The model under review builds one solid part; all positions refer to its coordinate system, in mm. Face numbers are marked on the shaded views. A direction names the side the tool comes from. Round coordinates to 2 decimals unless told otherwise and drop trailing zeros. Loops run counter-clockwise (first coordinate to the right, second up) from the corner with the lowest first, then second, coordinate; pieces in that order, holes last. Notation, with made-up numbers: M 29,72.5 L 68,72.5 A25 cw 68,93.5 Z; hole C 0.25,45.25 d6. An arc over 180 degrees is marked long. Answer in a Markdown table with one row per item. Add a question column.
from build123d import *

# Parameters (mm, degrees)
SKETCH1_W           = 29
SKETCH1_H           = 13
BOSS_EXTRUDE1_DEPTH = 19.92
SKETCH2_W           = 39.8
SKETCH2_H           = 13
SKETCH2_R           = 2
BOSS_EXTRUDE2_DEPTH = 3
SKETCH3_W           = 29
SKETCH3_H           = 13
BOSS_EXTRUDE3_DEPTH = 6.88
SKETCH4_R           = 6.5
BOSS_EXTRUDE4_DEPTH = 0.92
SKETCH5_R           = 2
BOSS_EXTRUDE5_DEPTH = 3.67


with BuildPart() as part:
    # Sketch1 → Boss-Extrude1 (new body)
    with BuildSketch(Plane(origin=(0, 0, 0), x_dir=(1, 0, 0), z_dir=(0, 1, 0))):
        with Locations((14.5, 6.5)):
            Rectangle(SKETCH1_W, SKETCH1_H)
    extrude(amount=BOSS_EXTRUDE1_DEPTH)

    # Sketch2 → Boss-Extrude2 (add)
    with BuildSketch(Plane(origin=(0, 19.92, 0), x_dir=(1, 0, 0), z_dir=(0, 1, 0))):
        with Locations((14.5, 6.5)):
            Rectangle(SKETCH2_W, SKETCH2_H)
        with Locations(Location((-3.05, 6.5, 0), (0, 0, 270))):
            Circle(SKETCH2_R, mode=Mode.SUBTRACT)
        with Locations(Location((32.05, 6.5, 0), (0, 0, 270))):
            Circle(SKETCH2_R, mode=Mode.SUBTRACT)
    extrude(amount=BOSS_EXTRUDE2_DEPTH)

    # Sketch3 → Boss-Extrude3 (add)
    with BuildSketch(Plane(origin=(0, 22.92, 0), x_dir=(1, 0, 0), z_dir=(0, 1, 0))):
        with Locations((14.5, 6.5)):
            Rectangle(SKETCH3_W, SKETCH3_H)
    extrude(amount=BOSS_EXTRUDE3_DEPTH)

    # Sketch4 → Boss-Extrude4 (add)
    with BuildSketch(Plane(origin=(0, 29.8, 0), x_dir=(1, 0, 0), z_dir=(0, 1, 0))):
        with Locations((22.5, 6.452760886)):
            Circle(SKETCH4_R)
    extrude(amount=BOSS_EXTRUDE4_DEPTH)

    # Sketch5 → Boss-Extrude5 (add)
    with BuildSketch(Plane(origin=(0, 30.72, 0), x_dir=(1, 0, 0), z_dir=(0, 1, 0))):
        with Locations(Location((22.5, 6.452760886, 0), (0, 0, 90))):
            Circle(SKETCH5_R)
    extrude(amount=BOSS_EXTRUDE5_DEPTH)


solid = part.part
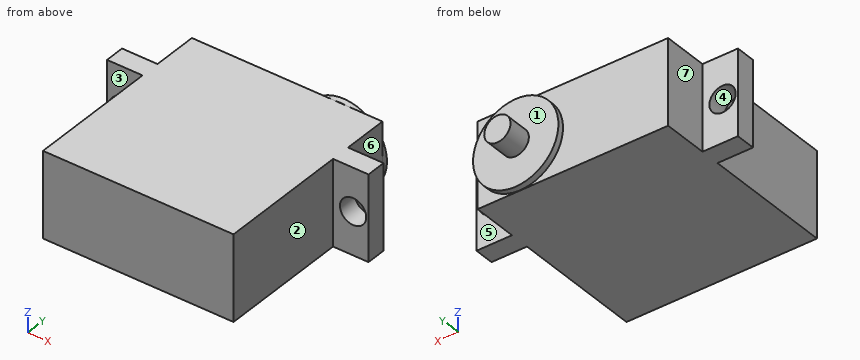
1. Take a section at D-D, the plane y = 26. State the section outline as (x, z) points, and give its area (3 significant figures).
2. Take a section at B-B, the plane z = -6. State how many separate pieces and enclosed holes the cut face has, and give its area (3 significant figures).
3. Take a section at A-A, the plane x = -3.05. State the section outline as (y, z) points.
4. For pin 1 Ø4 at (x, z) = (13, -4.5) entering from +Y; pin 2 Ø1.7 at (x, z) = (27, -3.5) entering from +Y; pin 3 Ø3 at (x, z) = (32.05, -6.5) entering from -Y; pin 4 Ø3.5 at (y, z) = (27.5, -7) entering from -X, all flat-tipped, find the tip position at first contact; note any pin that passes through.
5. Take a section at C-C, the plane x = 22.5. State the section outline as (y, z) points, and give its area (3 significant figures).
6. Machinability: for the marked faces 1, 2 and 3, which of the approach directions +Z, -Z, +X, -X, +Y, -Y give a long, thin tool a straight path to every point of the face, cutting with its end or side? Answer none if there is none.
7. Mouldability with a two-part tool opening along X and no side actions: class the marked faces 4, 5, 6 and 7 as released by +X, released by -X, zero draft, split by the parting line, or undercut.
8. To check wall thickness, follow probe 1 along X at (y, z) = (20.7, -6.5); probe 2 along Z at (x, y) = (-3, 21); probe 3 along X at (y, z) = (22, -8). State the ranges of each line that lie inside material, in increasing order.
Check sheet entries:
| question | item | result |
|---|---|---|
| 1 | outline | M 0,-13 L 29,-13 L 29,0 L 0,0 Z |
| 1 | area | 377 mm^2 |
| 2 | separate pieces | 3 |
| 2 | enclosed holes | 0 |
| 2 | area | 900 mm^2 |
| 3 | outline | M 19.92,-13 L 22.92,-13 L 22.92,-8.5 L 19.92,-8.5 Z; M 19.92,-4.5 L 22.92,-4.5 L 22.92,0 L 19.92,0 Z |
| 4 | pin 1 | stops at y = 29.8 |
| 4 | pin 2 | stops at y = 30.72 |
| 4 | pin 3 | passes through |
| 4 | pin 4 | stops at x = 0 |
| 5 | outline | M 0,-13 L 29.8,-13 L 29.8,-12.95 L 30.72,-12.95 L 30.72,-8.45 L 34.39,-8.45 L 34.39,-4.45 L 30.72,-4.45 L 30.72,0.05 L 29.8,0.05 L 29.8,0 L 0,0 Z |
| 5 | area | 414 mm^2 |
| 6 | face 1 | +Y |
| 6 | face 2 | +Z, -Z, +X, -Y |
| 6 | face 3 | +Z, -Z, -X, -Y |
| 7 | face 4 | undercut |
| 7 | face 5 | zero draft |
| 7 | face 6 | released by +X |
| 7 | face 7 | released by -X |
| 8 | probe 1 | x = -5.4 to -5.05, -1.05 to 30.05, 34.05 to 34.4 |
| 8 | probe 2 | z = -13 to -8.5, -4.5 to 0 |
| 8 | probe 3 | x = -5.4 to -4.37, -1.73 to 30.73, 33.37 to 34.4 |
